Source: CAD feature listing. Evaluate the final solid. Frame: model axes, mm. Face numbers are marked on the shaded views. Coordinates: 2 decimals unless noted, no trailing zeros. Order: outer loops, then holes, each group sorted by start corner. A loop starts at its lowest first (then second) coordinate and runs counter-clockwise, first axis right, second up. Notation, with made-up numbers: (-14.5, -35) - (32.5, -35) arc R24 ccw to (32.5, -10) - close; hole circle Ø5 at (37.25, 11.25). An arc over 180 degrees is marked (long way). One line per question, with ' | ' between items.
from build123d import *

# Parameters (mm, degrees)
CROQUIS1_R              = 0.5
SALIENTE_EXTRUIR1_DEPTH = 1.5
CROQUIS2_R              = 3.5
CROQUIS2_R_2            = 2.25
SALIENTE_EXTRUIR2_DEPTH = 2.5
CROQUIS3_R              = 2.5
CORTAR_EXTRUIR1_DEPTH   = 1
CROQUIS4_R              = 1
CORTAR_EXTRUIR2_DEPTH   = 1


with BuildPart() as part:
    # Croquis1 → Saliente-Extruir1 (new body)
    with BuildSketch(Plane(origin=(0, 0, 0), x_dir=(1, 0, 0), z_dir=(0, 1, 0))):
        with BuildLine():
            Line((-3.425882353, -0.716470588), (-2, -14.5))
            ThreePointArc((-2, -14.5), (0, -16.5), (2, -14.5))
            Line((2, -14.5), (3.425882353, -0.716470588))
            ThreePointArc((3.425882353, -0.716470588), (3.5, 0), (3.425882353, 0.716470588))
            Line((3.425882353, 0.716470588), (2, 14.5))
            ThreePointArc((2, 14.5), (0, 16.5), (-2, 14.5))
            Line((-2, 14.5), (-3.425882353, 0.716470588))
            ThreePointArc((-3.425882353, 0.716470588), (-3.5, 0), (-3.425882353, -0.716470588))
        make_face()
        with Locations(Location((0, -14.5, 0), (0, 0, 270))):
            Circle(CROQUIS1_R, mode=Mode.SUBTRACT)
        with Locations(Location((0, -12.5, 0), (0, 0, 270))):
            Circle(CROQUIS1_R, mode=Mode.SUBTRACT)
        with Locations(Location((0, -10.5, 0), (0, 0, 270))):
            Circle(CROQUIS1_R, mode=Mode.SUBTRACT)
        with Locations(Location((0, -8.5, 0), (0, 0, 270))):
            Circle(CROQUIS1_R, mode=Mode.SUBTRACT)
        with Locations(Location((0, -6.5, 0), (0, 0, 270))):
            Circle(CROQUIS1_R, mode=Mode.SUBTRACT)
        with Locations(Location((0, -4.5, 0), (0, 0, 270))):
            Circle(CROQUIS1_R, mode=Mode.SUBTRACT)
        with Locations(Location((0, 14.5, 0), (0, 0, 270))):
            Circle(CROQUIS1_R, mode=Mode.SUBTRACT)
        with Locations(Location((0, 12.5, 0), (0, 0, 270))):
            Circle(CROQUIS1_R, mode=Mode.SUBTRACT)
        with Locations(Location((0, 10.5, 0), (0, 0, 270))):
            Circle(CROQUIS1_R, mode=Mode.SUBTRACT)
        with Locations(Location((0, 8.5, 0), (0, 0, 270))):
            Circle(CROQUIS1_R, mode=Mode.SUBTRACT)
        with Locations(Location((0, 6.5, 0), (0, 0, 270))):
            Circle(CROQUIS1_R, mode=Mode.SUBTRACT)
        with Locations(Location((0, 4.5, 0), (0, 0, 270))):
            Circle(CROQUIS1_R, mode=Mode.SUBTRACT)
    extrude(amount=SALIENTE_EXTRUIR1_DEPTH)

    # Croquis2 → Saliente-Extruir2 (add)
    with BuildSketch(Plane(origin=(0, 1.5, 0), x_dir=(1, 0, 0), z_dir=(0, 1, 0))):
        with Locations(Location((0, 0, 0), (0, 0, 11.812282228))):
            Circle(CROQUIS2_R)
        with Locations(Location((0, 0, 0), (0, 0, 270))):
            Circle(CROQUIS2_R_2, mode=Mode.SUBTRACT)
    extrude(amount=SALIENTE_EXTRUIR2_DEPTH)

    # Croquis3 → Cortar-Extruir1 (cut)
    with BuildSketch(Plane.XZ):
        with Locations(Location((0, 0, 0), (0, 0, 270))):
            Circle(CROQUIS3_R)
    extrude(amount=-CORTAR_EXTRUIR1_DEPTH, mode=Mode.SUBTRACT)

    # Croquis4 → Cortar-Extruir2 (cut)
    with BuildSketch(Plane(origin=(0, 1.5, 0), x_dir=(1, 0, 0), z_dir=(0, 1, 0))):
        with Locations(Location((0, 0, 0), (0, 0, 270))):
            Circle(CROQUIS4_R)
    extrude(amount=-CORTAR_EXTRUIR2_DEPTH, mode=Mode.SUBTRACT)


solid = part.part
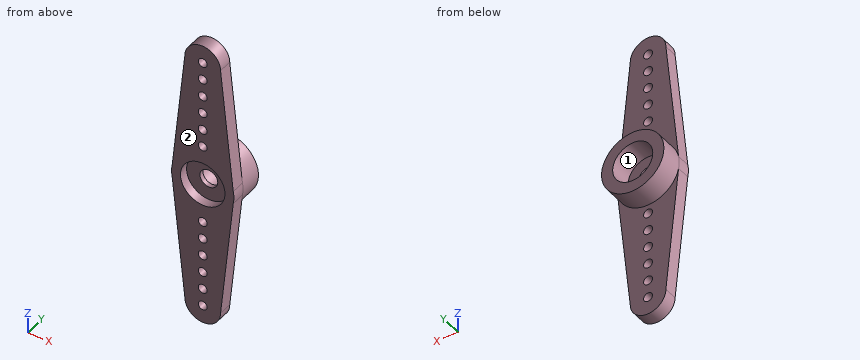
(1) Material intervals for L1, parallel to Y at x = 1, z = 6; L2, parallel to X at y = 1.2, z = 6.5; L3, parallel to Z at x = -0.25, y = 2.65, sorted ascending. Write a range as from..to.
Taken from the geometry:
L1: y = 0..1.5 | L2: x = -2.83..-0.5, 0.5..2.83 | L3: z = -3.49..-2.24, 2.24..3.49
(2) Cut plane D-D (y = 3.65). Return the cut outline in (x, z).
Taken from the geometry:
outline: circle Ø7 at (0, 0); hole circle Ø4.5 at (0, 0)
(3) Cut plane C-C (z = -10.5). Return the cut outline in (x, y), and give its area (3 significant figures).
Taken from the geometry:
outline: (-2.41, 0) - (-0.5, 0) - (-0.5, 1.5) - (-2.41, 1.5) - close; (0.5, 0) - (2.41, 0) - (2.41, 1.5) - (0.5, 1.5) - close | area: 5.74 mm²
(4) Pin query (flat end, axial travel): P1, Ø3.5, axis at x = 0, z = -1, coming from the +Y side; P2, Ø1, axis at x = 1, z = 0, coming from the -Y side; P3, Ø4, axis at x = 0, z = 0, coming from the +Y side. Return the tip coordinate at first contact, or that it passes through.
Taken from the geometry:
P1: stops at y = 4 | P2: stops at y = 1 | P3: stops at y = 1.5
(5) Pull-direction query (Z, two-part tool) for the marked faces 1 and 2; classes: pulls with the +Z half, pulls with the -Z half, needs draft (parallel to the pull), parting line crosses it, or undercut.
Taken from the geometry:
face 1: undercut | face 2: needs draft
(6) Cut plane A-A (z = 0). Return the cut outline in (x, y).
Taken from the geometry:
outline: (-3.5, 0) - (-2.5, 0) - (-2.5, 1) - (-1, 1) - (-1, 1.5) - (-2.25, 1.5) - (-2.25, 4) - (-3.5, 4) - close; (1, 1) - (2.5, 1) - (2.5, 0) - (3.5, 0) - (3.5, 4) - (2.25, 4) - (2.25, 1.5) - (1, 1.5) - close
(7) Cut plane B-B (x = 0). State how many separate pieces and enclosed holes the cut face has, and give its area (4 significant figures).
Taken from the geometry:
separate pieces: 14 | enclosed holes: 0 | area: 31.75 mm²
